Part model, mm, in its own coordinate system. A direction names the side the tool comes from. Give positions to 0.01 mm unless a question says otherwise; leave off trailing zeros. Write each loop counter-clockwise with the first axis right and the second up, starting at its lowest first coordinate (ties: lowest second). Pieces come first, ordered by that corner, then holes. Notation, with made-up numbers: (83.25, 9.5) - (90.25, 9.5) arc R27 cw to (90.25, 44.5) - close; hole circle Ø6 at (40, 54). An arc over 180 degrees is marked (long way). Answer as a JSON object with one key per item and string values. Group by question number.
```python
from build123d import *

# Parameters (mm, degrees)
SKETCH_1_W          = 43
SKETCH_1_H          = 7.5
EXTRUDE_1_DEPTH     = 1.5
SKETCH_2_R          = 1.65
CUT_EXTRUDE_2_DEPTH = 11.5
FILLET_1_R          = 3.75
SKETCH_3_W          = 30
SKETCH_3_H          = 14
EXTRUDE_3_DEPTH     = 1.5
SKETCH_4_W          = 15
SKETCH_4_H          = 32
EXTRUDE_4_DEPTH     = 3.25
SKETCH_5_R          = 2.1
CUT_EXTRUDE_3_DEPTH = 13
FILLET_3_R          = 5


with BuildPart() as part:
    # 草圖1 → 填料-伸長1 (new body)
    with BuildSketch(Plane(origin=(0, 0, 0), x_dir=(0, 0, -1), z_dir=(1, 0, 0))):
        Rectangle(SKETCH_1_W, SKETCH_1_H)
    extrude(amount=EXTRUDE_1_DEPTH)

    # 草圖2 → 除料-伸長2 (cut)
    with BuildSketch(Plane(origin=(1.5, 0, 0), x_dir=(0, 0, -1), z_dir=(1, 0, 0))):
        with Locations((-18.5, 0)):
            Circle(SKETCH_2_R)
        with Locations((18.5, 0)):
            Circle(SKETCH_2_R)
    extrude(amount=-CUT_EXTRUDE_2_DEPTH, mode=Mode.SUBTRACT)

    # 圓角1
    fillet_1_edges = [part.edges().sort_by_distance(p)[0] for p in [
        (0.75, -3.75, -21.5),
        (0.75, 3.75, -21.5),
        (0.75, -3.75, 21.5),
        (0.75, 3.75, 21.5),
    ]]
    fillet(fillet_1_edges, radius=FILLET_1_R - 0.0001)  # a hair under: the kernel refuses the full size

    # 草圖3 → 填料-伸長3 (add)
    with BuildSketch(Plane.ZY):
        Rectangle(SKETCH_3_W, SKETCH_3_H)
    extrude(amount=-EXTRUDE_3_DEPTH)

    # 草圖4 → 填料-伸長4 (add)
    with BuildSketch(Plane(origin=(0, 7, 0), x_dir=(1, 0, 0), z_dir=(0, 1, 0))):
        with Locations((7.5, 0)):
            Rectangle(SKETCH_4_W, SKETCH_4_H)
    extrude(amount=-EXTRUDE_4_DEPTH)

    # 草圖5 → 除料-伸長3 (cut)
    with BuildSketch(Plane.XZ.offset(-3.75)):
        with Locations(Location((7.9, 12, 0), (0, 0, 270))):
            Circle(SKETCH_5_R)
        with Locations(Location((7.9, 4, 0), (0, 0, 270))):
            Circle(SKETCH_5_R)
        with Locations(Location((7.9, -4, 0), (0, 0, 270))):
            Circle(SKETCH_5_R)
        with Locations(Location((7.9, -12, 0), (0, 0, 270))):
            Circle(SKETCH_5_R)
    extrude(amount=-CUT_EXTRUDE_3_DEPTH, mode=Mode.SUBTRACT)

    # 圓角3
    fillet_3_edges = [part.edges().sort_by_distance(p)[0] for p in [
        (15, 5.375, -16),
        (15, 5.375, 16),
    ]]
    fillet(fillet_3_edges, radius=FILLET_3_R)


solid = part.part
```
1) Band-saw the part on D-D (z = -1.5). List the corners of the cut face in (x, y).
2) Probe line 1 (X direction, y = 5.5, z = -4); line 2 (X direction, y = 2.25, z = -3); line 3 (Y direction, x = 11.25, z = -6). List the from-to ranges inside material, lowest first.
3) Band-saw the part on B-B (y = 4.5). List the corners of the cut face in (x, z), plus the area to 3 significant figures.
4) Which spindle directions (+Z, -Z, +X, -X, +Y, -Y) get a long thin tool onto all of the face, cutting with end or side? Do faces 1 (the flat face through (8, 3.75, 0)), 2 (the flat face through (1, 3.75, 17)), 3 (the flat face through (1, -3.75, -16)), 4 (the flat face through (1, -5, 15)). Say none if no direction does.
5) Drop flat-ended pins along their axis: P1, Ø0.8, axis at x = 0.5, z = -16.5, coming from the -Y side; P2, Ø3, axis at y = 3.5, z = -17, coming from the +X side; P3, Ø6.5, axis at x = 7.9, z = -4, coming from the -Y side. Give the stop position or say it passes through.
6) Band-saw the part on A-A (z = 4). List the corners of the cut face in (x, y), plus the area to 3 significant figures.
7) Band-saw the part on C-C (y = 0.5). List the corners of the cut face in (x, z), plus the area to 3 significant figures.
8) Mould opens along X. For faces 5 (the flat face through (1, -5, -15)), 6 (the cylindrical face through (5.85, 5.35, 4.46)), 7 (the flat face through (1.5, -2, 0)) say: pulls with the +X half, pulls with the -X half, needs draft (parallel to the pull), parting line crosses it, or undercut.
Verdict:
{
 "1": {"outline": "(0, -7) - (1.5, -7) - (1.5, 3.75) - (15, 3.75) - (15, 7) - (0, 7) - close"},
 "2": {"line 1": "0 to 5.8, 10 to 15", "line 2": "0 to 1.5", "line 3": "3.75 to 7"},
 "3": {"outline": "(0, -16) - (10, -16) arc R5 ccw to (15, -11) - (15, 11) arc R5 ccw to (10, 16) - (0, 16) - close; hole circle Ø4.2 at (7.9, -12); hole circle Ø4.2 at (7.9, -4); hole circle Ø4.2 at (7.9, 4); hole circle Ø4.2 at (7.9, 12)", "area": "414 mm2"},
 "4": {"face 1": "+Z, -Z, +X, -Y", "face 2": "+Z, +X, -X, +Y", "face 3": "-Z, +X, -X, -Y", "face 4": "+Z, +X, -X, -Y"},
 "5": {"P1": "y = -3.75", "P2": "x = 12.14", "P3": "y = 3.75"},
 "6": {"outline": "(0, -7) - (1.5, -7) - (1.5, 3.75) - (5.8, 3.75) - (5.8, 7) - (0, 7) - close; (10, 3.75) - (15, 3.75) - (15, 7) - (10, 7) - close", "area": "51.2 mm2"},
 "7": {"outline": "(0, -21.47) - (1.5, -21.47) - (1.5, -20.07) - (0, -20.07) - close; (0, -16.93) - (1.5, -16.93) - (1.5, 16.93) - (0, 16.93) - close; (0, 20.07) - (1.5, 20.07) - (1.5, 21.47) - (0, 21.47) - close", "area": "55.0 mm2"},
 "8": {"face 5": "needs draft", "face 6": "undercut", "face 7": "pulls with the +X half"}
}
